from build123d import *

# Parameters (mm, degrees)
SKETCH1_R               = 3
BOSS_EXTRUDE1_DEPTH     = 60
SKETCH2_R               = 6
BOSS_EXTRUDE2_DEPTH     = 3
SKETCH3_R               = 1.5
CUT_EXTRUDE1_DEPTH      = 7
CUT_EXTRUDE1_DEPTH_BACK = 7


with BuildPart() as part:
    # Sketch1 → Boss-Extrude1 (new body)
    with BuildSketch(Plane(origin=(0, 0, 0), x_dir=(0, 0, -1), z_dir=(1, 0, 0))):
        Circle(SKETCH1_R)
    extrude(amount=BOSS_EXTRUDE1_DEPTH)

    # Sketch2 → Boss-Extrude2 (add)
    with BuildSketch(Plane(origin=(60, 0, 0), x_dir=(0, 0, -1), z_dir=(1, 0, 0))):
        Circle(SKETCH2_R)
    extrude(amount=BOSS_EXTRUDE2_DEPTH)

    # Sketch3 → Cut-Extrude1 (cut, two sides)
    with BuildSketch(Plane.XY) as cut_extrude1_sk:
        with Locations((4, 0)):
            Circle(SKETCH3_R)
    extrude(amount=CUT_EXTRUDE1_DEPTH, mode=Mode.SUBTRACT)
    extrude(cut_extrude1_sk.sketch, amount=-CUT_EXTRUDE1_DEPTH_BACK, mode=Mode.SUBTRACT)


solid = part.part
Verification items for the finished model (mm, model axes). A direction names the side the tool comes from. Coordinates: 2 decimals unless noted, no trailing zeros. Order: outer loops, then holes, each group sorted by start corner. A loop starts at its lowest first (then second) coordinate and runs counter-clockwise, first axis right, second up.
1. Sectioned sample at A-A, the plane y = 0. Record the cut outline in (x, z).
Results found:
outline: (0, -3) - (2.5, -3) - (2.5, 3) - (0, 3) - close; (5.5, -3) - (60, -3) - (60, -6) - (63, -6) - (63, 6) - (60, 6) - (60, 3) - (5.5, 3) - close
2. Sectioned sample at C-C, the plane x = 4. Record the cut outline in (y, z).
Results found:
outline: (-1.5, -2.6) - (-1.5, 2.6) arc R3 ccw to start; (1.5, -2.6) arc R3 ccw to (1.5, 2.6) - close
3. Sectioned sample at B-B, the plane z = 0. Record the cut outline in (x, y).
Results found:
outline: (0, -3) - (60, -3) - (60, -6) - (63, -6) - (63, 6) - (60, 6) - (60, 3) - (0, 3) - close; hole circle Ø3 at (4, 0)
4. Set-up check for faces 1 (the face through (60, -1, 3)), 2 (the face through (63, 0, 0)): record each of +Z, -Z, +X, -X, +Y, -Y from which the full face is reachable in a straight line by a thin tool's end or side.
Results found:
face 1: -X
face 2: +Z, -Z, +X, +Y, -Y
5. Release check for a two-part mould opening along X. For faces 3 (the face through (61, 0, 6)), 4 (the face through (0, 0, 0)), 5 (the face through (4.806, 1.265, 0.042)) record: +X half, -X half, draft (parallel to the pull), parting line (faces both ways), or undercut.
Results found:
face 3: draft
face 4: -X half
face 5: undercut
6. Scan lines: line 1 (X direction, y = 0, z = -1); line 2 (Y direction, x = 4, z = 0.25); line 3 (X direction, y = 5.25, z = -1.5). Record each from-to range of solid material in increasing order.
Results found:
line 1: x = 0 to 2.5, 5.5 to 63
line 2: y = -2.99 to -1.5, 1.5 to 2.99
line 3: x = 60 to 63
7. Go/stop test with flat-tipped pins: pin 1 Ø5 at (x, y) = (17.5, 0.5) entering from +Z; pin 2 Ø3.5 at (x, y) = (4, 0) entering from -Z. Record where each tip stops, or that it passes through.
Results found:
pin 1: stops at z = 3
pin 2: stops at z = -3
8. Sectioned sample at D-D, the plane x = 13. Record the cut outline in (y, z), and give its area (3 significant figures).
Results found:
outline: circle Ø6 at (0, 0)
area: 28.3 mm2
